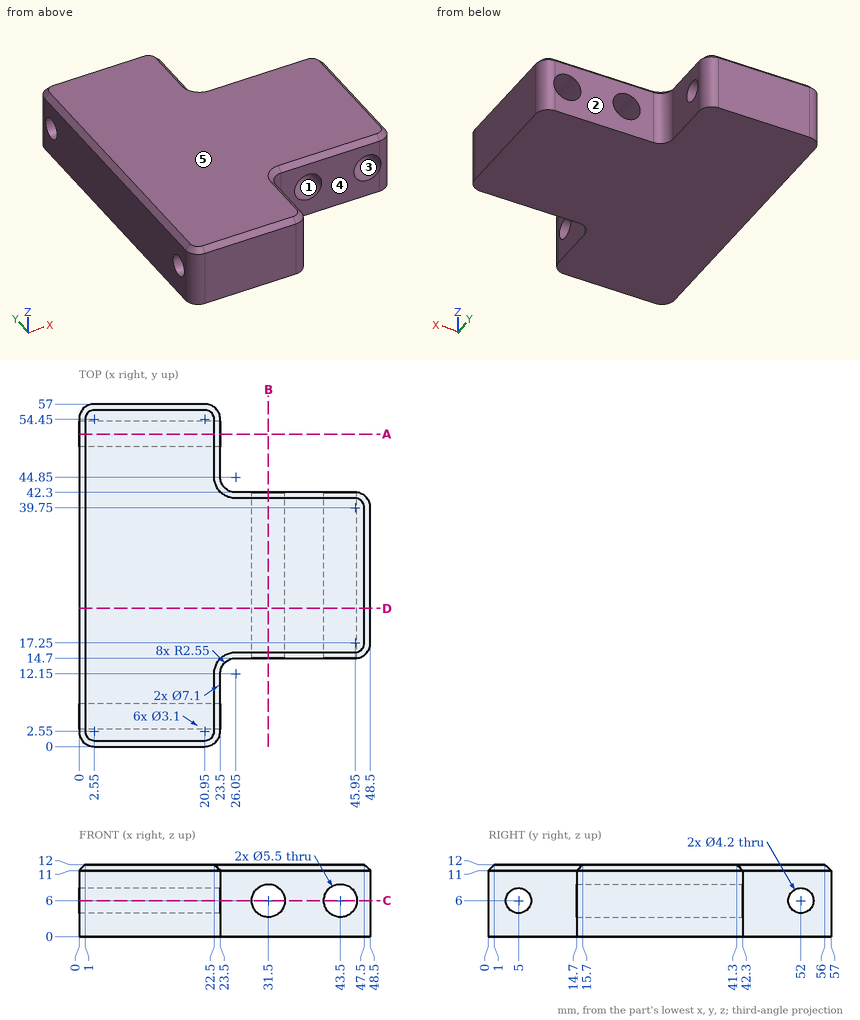
Design review of the part shown in the three views and the two pictorial views. Dimensions are in mm from the part's minimum x, y and z. A direction names the side the tool comes from. Round coordinates to 2 decimals unless told otherwise and drop trailing zeros. Loops run counter-clockwise (first coordinate to the right, second up) from the corner with the lowest first, then second, coordinate; pieces in that order, holes last. Notation, with made-up numbers: M 8.25,77 L 37.25,77 A7 ccw 37.25,83 Z; hole C 41,0 d8. An arc over 180 degrees is marked long. Answer as a JSON object with one key per item and string values.
Item 1: Wall thickness on L1, parallel to Y at x = 15, z = 6; L2, parallel to X at y = 32, z = 6.25; L3, parallel to X at y = 28, z = 5.25: over which ranges is each line inside the solid? List them lowest first. Write a range as from..to.
Answer sheet:
{"L1": "y = 0..2.9, 7.1..49.9, 54.1..57", "L2": "x = 0..28.76, 34.24..40.76, 46.24..48.5", "L3": "x = 0..28.85, 34.15..40.85, 46.15..48.5"}
Item 2: We need section B-B on x = 31.5. Give the boundary of the cut face in (y, z), and give its area (3 significant figures).
Answer sheet:
{"outline": "M 14.7,0 L 42.3,0 L 42.3,3.25 L 14.7,3.25 Z; M 14.7,8.75 L 42.3,8.75 L 42.3,11 L 41.3,12 L 15.7,12 L 14.7,11 Z", "area": "178 mm^2"}
Item 3: We need section C-C on z = 6. State how many separate pieces and enclosed holes the cut face has, and give its area (3 significant figures).
Answer sheet:
{"separate pieces": "5", "enclosed holes": "0", "area": "1,520 mm^2"}
Item 4: We need section A-A on y = 52. Give the boundary of the cut face in (x, z), and give its area (3 significant figures).
Answer sheet:
{"outline": "M 0,0 L 23.5,0 L 23.5,3.9 L 0,3.9 Z; M 0,8.1 L 23.5,8.1 L 23.5,11 L 22.5,12 L 1,12 L 0,11 Z", "area": "182 mm^2"}
Item 5: Clearance check with flat-ended pins moving along their axes: P1, Ø6.5, axis at x = 43.5, z = 6, coming from the +Y side; P2, Ø5, axis at y = 9, z = 6.5, coming from the +X side. State where each tip first meets the part, or that it passes through.
Answer sheet:
{"P1": "stops at y = 42.3", "P2": "stops at x = 23.5"}
Item 6: Machinability: for the marked faces 1 and 2, which of the approach directions +Z, -Z, +X, -X, +Y, -Y give a long, thin tool a straight path to every point of the face, cutting with its end or side? Answer none if there is none.
Answer sheet:
{"face 1": "+Y, -Y", "face 2": "+Z, -Z, +X, +Y"}
Item 7: The part is to be moulded in two halves that separate along Z. For the marked faces 3, 4 and 5, say which applies: pulls with the +Z half, pulls with the -Z half, needs draft (parallel to the pull), parting line crosses it, or undercut.
Answer sheet:
{"face 3": "undercut", "face 4": "needs draft", "face 5": "pulls with the +Z half"}
Item 8: We need section D-D on y = 23. Give the boundary of the cut face in (x, z), and give its area (3 significant figures).
Answer sheet:
{"outline": "M 0,0 L 48.5,0 L 48.5,11 L 47.5,12 L 1,12 L 0,11 Z; hole C 31.5,6 d5.5; hole C 43.5,6 d5.5", "area": "533 mm^2"}
